Part model, mm, in its own coordinate system. A direction names the side the tool comes from. Round coordinates to 2 decimals unless told otherwise and drop trailing zeros. Loops run counter-clockwise (first coordinate to the right, second up) from the corner with the lowest first, then second, coordinate; pieces in that order, holes last. Notation, with made-up numbers: M 87.25,65.25 L 109.25,65.25 A17 ccw 109.25,69.25 Z; hole C 2,-24.75 d5. An arc over 180 degrees is marked long. Put each result on its own line as item: value. Start each with the question number.
1) Which spindle directions (+Z, -Z, +X, -X, +Y, -Y) get a long thin tool onto all of the face, cutting with end or side? Do faces 4 (the cylindrical face through (23.846, -65.554, 7.509)), 5 (the flat face through (0, 0, 0)). Say none if no direction does.
2) Slice it at B-B on z = 0. Give the cut face in (x, y), then the cut area to 3 significant figures.
3) Pull direction X, two halves, no side cores. Call faces 1 (the flat face through (6, -130, -27)), 2 (the flat face through (0, -5, 0)), 3 (the cylindrical face through (-29.97, -63.02, 1.32)): +X half, -X half, draft (parallel to the pull), parting line (faces both ways), or undercut.
4) Drop flat-ended pins along their axis: pin 1 Ø5 at (x, z) = (-19, -11.5) entering from -Y; pin 2 Ø1 at (x, y) = (20.5, -40) entering from -Z; pin 3 Ø12 at (x, y) = (22.5, -76) entering from +Z. Give the stop position or say it passes through.
5) Probe line 1 along Z through (x, y) = (0, -59); line 2 along Z through (x, y) = (6.5, -13); line 3 along X through (y, z) = (-93, -22.5). List the from-to ranges inside material, lowest first.
6) Slice it at C-C on x = 0. Give the cut face in (y, z).
7) Slice it at A-A on y = -75.5. Give the cut face in (x, z).
```python
from build123d import *

# Parameters (mm, degrees)
F0_R     = 30
F0_R_2   = 25
F1_DEPTH = 5
F2_DEPTH = 130
F3_R     = 2.172792
F4_R     = 2.172792


with BuildPart() as f1:
    # F0 (on Front) → F1 (new body)
    with BuildSketch(Plane.XZ):
        Circle(F0_R)
        Circle(F0_R_2, mode=Mode.SUBTRACT)
        Circle(F0_R_2)
    extrude(amount=F1_DEPTH)

    # F0 (on Front) → F2 (join)
    with BuildSketch(Plane.XZ):
        Circle(F0_R)
        Circle(F0_R_2, mode=Mode.SUBTRACT)
    extrude(amount=F2_DEPTH)

    # F3
    f3_edges = [f1.edges().sort_by_distance(p)[0] for p in [
        (-30, -130, 0),
    ]]
    fillet(f3_edges, radius=F3_R)

    # F4
    f4_edges = [f1.edges().sort_by_distance(p)[0] for p in [
        (-25, -130, 0),
    ]]
    fillet(f4_edges, radius=F4_R)


solid = f1.part
```
Recorded:
1. face 4: -Y
1. face 5: +Z, -Z, +X, -X, +Y
2. outline: M -30,-127.83 A2.17 ccw -27.83,-130 L -27.17,-130 A2.17 ccw -25,-127.83 L -25,-5 L 25,-5 L 25,-127.83 A2.17 ccw 27.17,-130 L 27.83,-130 A2.17 ccw 30,-127.83 L 30,0 L -30,0 Z
2. area: 1,550 mm2
3. face 1: draft
3. face 2: undercut
3. face 3: parting line
4. pin 1: stops at y = -5
4. pin 2: stops at z = -22.36
4. pin 3: stops at z = 25.05
5. line 1: z = -30 to -25, 25 to 30
5. line 2: z = -29.29 to -24.14, 24.14 to 29.29
5. line 3: x = -19.84 to -10.9, 10.9 to 19.84
6. outline: M -130,-27.83 A2.17 ccw -127.83,-30 L 0,-30 L 0,30 L -127.83,30 A2.17 ccw -130,27.83 L -130,27.17 A2.17 ccw -127.83,25 L -5,25 L -5,-25 L -127.83,-25 A2.17 ccw -130,-27.17 Z
7. outline: C 0,0 d60; hole C 0,0 d50
